Autodesk Inventor part; units mm, degrees
ref_plane "YZ Plane" through (0, 0, 0) normal (1, 0, 0) x (0, 1, 0)
ref_plane "XZ Plane" through (0, 0, 0) normal (0, 1, 0) x (-1, 0, 0)
ref_plane "XY Plane" through (0, 0, 0) normal (0, 0, 1) x (1, 0, 0)
sketch "Sketch1" plane through (0, 0, 0) normal (0, 0, 1) x (1, 0, 0)
  circle A0 centre (0, 0) radius 1.5
  circle A1 centre (-15, 0) radius 0.75
  line L0 (-15, 0) -> (0, 0) construction
  arc A2 (-0.4083, -3.4761) -> (-0.4083, 3.4761) centre (0, 0) ccw
  arc A3 (-15.2042, 1.738) -> (-15.2042, -1.738) centre (-15, 0) ccw
  circle A4 centre (-12, 0) radius 0.75
  circle A5 centre (-9, 0) radius 0.75
  line L1 (-15.2042, 1.738) -> (-0.4083, 3.4761)
  line L2 (-0.4083, -3.4761) -> (-15.2042, -1.738)
  dimension "d0" = 15
  dimension "d1" = 1.5
  dimension "d2" = 3
  dimension "d5" = 3
  dimension "d10" = 1
  dimension "d11" = 2
extrude "Extrusion1" add sketch "Sketch1" along normal blind 1
sketch "Sketch2" plane through (0, 0, 1) normal (0, 0, 1) x (1, 0, 0)
  arc A0 (-0.4083, -3.4761) -> (-0.4083, 3.4761) centre (0, 0) ccw
  circle A1 centre (0, 0) radius 3.5
  circle A2 centre (0, 0) radius 2.4727
  point P0 (-0.4083, -3.4761)
extrude "Extrusion2" add sketch "Sketch2" along normal blind 3
properties part number "ServoHorn"
Model file for the job. Use its own axes, mm. A direction names the side the tool comes from. Coordinates: 2 decimals unless noted, no trailing zeros. Order: outer loops, then holes, each group sorted by start corner. A loop starts at its lowest first (then second) coordinate and runs counter-clockwise, first axis right, second up. Notation, with made-up numbers: (-12.5, 50) - (39.5, 50) arc R22 cw to (39.5, 66) - close; hole circle Ø11 at (-37, 83.5). An arc over 180 degrees is marked (long way). Return JSON: item names as keys, results as strings. Group by question number.
1) Mould opens along Y. For faces 1 (the flat face through (-7.91, 2.595, 0.493)), 2 (the flat face through (-9, -1, 1)), 3 (the cylindrical face through (-15.75, -0.03, 0.49)) say: released by +Y, released by -Y, zero draft, split by the parting line, or undercut.
2) Saw through at C-C, the plane y = -1.25. Write the cut outline in (x, z), plus the area to 3 significant figures.
3) Tool access for faces 4 (the flat face through (0, -2, 1)), 5 (the flat face through (-7, 0, 0)): list every direction of +Z, -Z, +X, -X, +Y, -Y with a clear straight run to the whole face (end or side of a thin tool).
4) Saw through at D-D, the plane z = 3.6. Write the cut outline in (x, y), plus the area to 3 significant figures.
5) Probe line 1 (Y direction, x = 0, z = 3.2); line 2 (Z direction, x = -5.5, y = -1.5); line 3 (Y direction, x = 0, z = 0.3). List the from-to ranges inside material, lowest first. Write a range as from..to.
6) Saw through at B-B, the plane z = 0.75. Write the cut outline in (x, y), plus the area to 3 significant figures.
7) Flat gauge pin, fed straight in: P1, Ø1.7, axis at x = -15, y = 0, coming from the +Z side. Where does the tip first touch, or does it go through?
8) Saw through at A-A, the plane x = 0. Write the cut outline in (y, z).
Values found:
{
 "1": {"face 1": "released by +Y", "face 2": "zero draft", "face 3": "undercut"},
 "2": {"outline": "(-16.22, 0) - (-0.83, 0) - (-0.83, 1) - (-2.13, 1) - (-2.13, 4) - (-3.27, 4) - (-3.27, 1) - (-16.22, 1) - close; (0.83, 0) - (3.27, 0) - (3.27, 4) - (2.13, 4) - (2.13, 1) - (0.83, 1) - close", "area": "24.6 mm²"},
 "3": {"face 4": "+Z", "face 5": "-Z, +X, -X, +Y, -Y"},
 "4": {"outline": "(-0.41, -3.48) arc R3.5 ccw (long way) to (-0.41, 3.48) arc R3.5 ccw to start; hole circle Ø4.95 at (0, 0)", "area": "19.3 mm²"},
 "5": {"line 1": "y = -3.5..-2.47, 2.47..3.5", "line 2": "z = 0..1", "line 3": "y = -3.5..-1.5, 1.5..3.5"},
 "6": {"outline": "(-15.2, -1.74) - (-0.41, -3.48) arc R3.5 ccw (long way) to (-0.41, 3.48) - (-15.2, 1.74) arc R1.75 ccw to start; hole circle Ø1.5 at (-15, 0); hole circle Ø1.5 at (-12, 0); hole circle Ø1.5 at (-9, 0); hole circle Ø3 at (0, 0)", "area": "91.0 mm²"},
 "7": {"P1": "stops at z = 1"},
 "8": {"outline": "(-3.5, 0) - (-1.5, 0) - (-1.5, 1) - (-2.47, 1) - (-2.47, 4) - (-3.5, 4) - close; (1.5, 0) - (3.5, 0) - (3.5, 4) - (2.47, 4) - (2.47, 1) - (1.5, 1) - close"}
}
